Check sheet for the modelled part. Datum: model origin and axes. Units: mm. A direction names the side the tool comes from. Round coordinates to 2 decimals unless told otherwise and drop trailing zeros. Write each loop counter-clockwise with the first axis right and the second up, starting at its lowest first coordinate (ties: lowest second). Pieces come first, ordered by that corner, then holes. Notation, with made-up numbers: (-21, -23) -> (27, -23) arc R29 cw to (27, 16) -> close; hole circle Ø11 at (30, 8). An arc over 180 degrees is marked (long way). One line per item, written item: value.
from build123d import *

# Parameters (mm, degrees)
SKETCH_R      = 0.95
SKETCH_R_2    = 1.15
PAD_DEPTH     = 5
SKETCH001_R   = 3.8
SKETCH001_R_2 = 0.95
PAD001_DEPTH  = 5
FILLET_R      = 1


with BuildPart() as part:
    # Sketch → Pad (new body)
    with BuildSketch(Plane.XY):
        with BuildLine():
            ThreePointArc((-26.31583, -31.143856), (-24.856144, -36.31583), (-19.68417, -34.856144))
            Line((-19.68417, -34.856144), (-5.959198, -10.337748))
            Line((-5.959198, -10.337748), (0, -10.337748))
            Line((0, -10.337748), (0, 8.381557))
            Line((-5.959198, 8.381557), (0, 8.381557))
            Line((-19.626283, 34.748723), (-5.959198, 8.381557))
            ThreePointArc((-19.626283, 34.748723), (-24.755923, 36.369975), (-26.366218, 31.236885))
            Line((-26.366218, 31.236885), (-9.988881, -0.031456))
            Line((-9.988881, -0.031456), (-9.988881, -1.977268))
            Line((-9.988881, -1.977268), (-26.31583, -31.143856))
        make_face()
        with Locations((-23, 33)):
            Circle(SKETCH_R, mode=Mode.SUBTRACT)
        with Locations((-23, -33)):
            Circle(SKETCH_R, mode=Mode.SUBTRACT)
        with Locations((-13.8, 15.434951)):
            Circle(SKETCH_R_2, mode=Mode.SUBTRACT)
        with Locations((-13.8, -16.565049)):
            Circle(SKETCH_R_2, mode=Mode.SUBTRACT)
    extrude(amount=PAD_DEPTH)

    # Sketch001 (on Face16 of Pad) → Pad001 (join)
    with BuildSketch(Plane.XY.offset(5)):
        with Locations((-23, 33)):
            Circle(SKETCH001_R)
        with Locations((-23, 33)):
            Circle(SKETCH001_R_2, mode=Mode.SUBTRACT)
        with Locations((-23, -33)):
            Circle(SKETCH001_R)
        with Locations((-23, -33)):
            Circle(SKETCH001_R_2, mode=Mode.SUBTRACT)
    extrude(amount=PAD001_DEPTH)

    # Mirrored: part across Sketch001 V_Axis


with BuildPart() as part_1:
    add(part.part)
    add(part.part.mirror(Plane(origin=(0, 0, 5), x_dir=(0, 0, 1), z_dir=(1, 0, 0))))

    # Fillet
    fillet_edges = [part_1.edges().sort_by_distance(p)[0] for p in [
        (-5.959198, -10.337748, 2.5),
        (5.959198, -10.337748, 2.5),
        (-9.988881, -0.031456, 2.5),
        (-9.988881, -1.977268, 2.5),
        (-5.959198, 8.381557, 2.5),
        (5.959198, 8.381557, 2.5),
        (9.988881, -1.977268, 2.5),
        (9.988881, -0.031456, 2.5),
    ]]
    fillet(fillet_edges, radius=FILLET_R)


solid = part_1.part
Item 1: Depth check by flat-ended pin: P1, Ø6, axis at x = 17.5, z = 3, coming from the +Y side; P2, Ø1.2, axis at y = -1, z = 3, coming from the -X side; P3, Ø1.6, axis at y = -1, z = 3, coming from the +X side. Enter the tip coordinate at first touch or a pass-through.
Answer:
P1: stops at y = 35.86
P2: stops at x = -9.99
P3: stops at x = 9.99
Item 2: Sectioned sample at D-D on x = -23. Enter the section's corners in (y, z).
Answer:
outline: (-36.8, 0) -> (-33.95, 0) -> (-33.95, 10) -> (-36.8, 10) -> close; (-32.05, 0) -> (-25.22, 0) -> (-25.22, 5) -> (-29.2, 5) -> (-29.2, 10) -> (-32.05, 10) -> close; (24.81, 0) -> (32.05, 0) -> (32.05, 10) -> (29.2, 10) -> (29.2, 5) -> (24.81, 5) -> close; (33.95, 0) -> (36.8, 0) -> (36.8, 10) -> (33.95, 10) -> close
Item 3: Sectioned sample at B-B on x = 18. Enter the section's corners in (y, z).
Answer:
outline: (-31.85, 0) -> (-16.29, 0) -> (-16.29, 5) -> (-31.85, 5) -> close; (15.26, 0) -> (31.61, 0) -> (31.61, 5) -> (15.26, 5) -> close
Item 4: Tool access check on faces 5 (the cylindrical face through (13.3, -17.6, 2.5)), 6 (the flat face through (18.35, 15.93, 2.46)), 7 (the flat face through (0, 8.382, 2)), 8 (the flat face through (0, -10.338, 2)). Record the directions out of +Z, -Z, +X, -X, +Y, -Y that give a thin tool (end or side, any length) a straight path to the whole face; none if there is none.
Answer:
face 5: +Z, -Z
face 6: +Z, -Z, +X
face 7: +Z, -Z, +Y
face 8: +Z, -Z, -Y
Item 5: Mould release check, pull along Y, two halves, no side actions. Record for faces 1 (the flat face through (2, 0, 0)), 2 (the flat face through (13.06, -23.02, 2.46)), 3 (the flat face through (-18.35, 15.93, 2.46)), 4 (the cylindrical face through (22.56, -33.84, 4.93)): pulls with the +Y half, pulls with the -Y half, needs draft (parallel to the pull), parting line crosses it, or undercut.
Answer:
face 1: needs draft
face 2: pulls with the -Y half
face 3: undercut
face 4: undercut
Item 6: Sectioned sample at A-A on z = 6.5. Enter the section's corners in (x, y), and give its area (3 significant figures).
Answer:
outline: circle Ø7.6 at (-23, -33); circle Ø7.6 at (-23, 33); circle Ø7.6 at (23, -33); circle Ø7.6 at (23, 33); hole circle Ø1.9 at (-23, -33); hole circle Ø1.9 at (-23, 33); hole circle Ø1.9 at (23, -33); hole circle Ø1.9 at (23, 33)
area: 170 mm^2
Item 7: Sectioned sample at C-C on y = 33. Enter the section's corners in (x, z), and give its area (3 significant figures).
Answer:
outline: (-26.8, 0) -> (-23.95, 0) -> (-23.95, 10) -> (-26.8, 10) -> close; (-22.05, 0) -> (-18.72, 0) -> (-18.72, 5) -> (-19.2, 5) -> (-19.2, 10) -> (-22.05, 10) -> close; (18.72, 0) -> (22.05, 0) -> (22.05, 10) -> (19.2, 10) -> (19.2, 5) -> (18.72, 5) -> close; (23.95, 0) -> (26.8, 0) -> (26.8, 10) -> (23.95, 10) -> close
area: 119 mm^2
Item 8: Thickness scan on line 1 (Y direction, x = 23, z = 6); line 2 (X direction, y = -33, z = 6); line 3 (Y direction, x = -23, z = 4.5). Record the ranges inside material, lowest first.
Answer:
line 1: y = -36.8 to -33.95, -32.05 to -29.2, 29.2 to 32.05, 33.95 to 36.8
line 2: x = -26.8 to -23.95, -22.05 to -19.2, 19.2 to 22.05, 23.95 to 26.8
line 3: y = -36.8 to -33.95, -32.05 to -25.22, 24.81 to 32.05, 33.95 to 36.8
